```python
from build123d import *

# Parameters (mm, degrees)
SKETCH1_W                    = 125.73
SKETCH1_H                    = 76.2
BASE_FLANGE1_DEPTH           = 1.2192
EDGE_FLANGE1_STRIP_W         = 7.4168
EDGE_FLANGE1_STRIP_H         = 1.2192
EDGE_FLANGE1_STRIP_CUT_DEPTH = 76.2
EDGE_FLANGE1_DEPTH           = 76.2
EDGE_FLANGE2_STRIP_W         = 7.4168
EDGE_FLANGE2_STRIP_H         = 1.2192
EDGE_FLANGE2_STRIP_CUT_DEPTH = 123.2408
EDGE_FLANGE2_DEPTH           = 123.2408
EDGE_FLANGE3_STRIP_W         = 7.4168
EDGE_FLANGE3_STRIP_H         = 1.2192
EDGE_FLANGE3_STRIP_CUT_DEPTH = 200.7108
EDGE_FLANGE3_DEPTH           = 200.7108
BREAK_CORNER5_START          = -96.12466152
BREAK_CORNER5_OUTLINE_W      = 143.62455456
BREAK_CORNER5_OUTLINE_H      = 4
BREAK_CORNER5_DEPTH          = 7.220125921
BREAK_CORNER5_START_2        = 38.579180296
BREAK_CORNER5_2_OUTLINE_W    = 8.37544544
BREAK_CORNER5_2_OUTLINE_H    = 4
BREAK_CORNER5_2_DEPTH        = 14.440251843
BREAK_CORNER6_START          = -96.12466152
BREAK_CORNER6_OUTLINE_W      = 88.7601302
BREAK_CORNER6_OUTLINE_H      = 4
BREAK_CORNER6_DEPTH          = 7.220125921
BREAK_CORNER6_START_2        = -16.200382042
BREAK_CORNER6_2_OUTLINE_W    = 8.2398698
BREAK_CORNER6_2_OUTLINE_H    = 4
BREAK_CORNER6_2_DEPTH        = 14.440251842


# Read off the part's stored shape, not the designer's step: Break-Corner5, Break-Corner6
# Sheet-metal steps are written as plain solids
with BuildPart() as part:
    # Sketch1 → Base-Flange1 (new body)
    with BuildSketch(Plane(origin=(0, 0, 0), x_dir=(0, 0, -1), z_dir=(1, 0, 0))):
        with Locations((62.865, 38.1)):
            Rectangle(SKETCH1_W, SKETCH1_H)
    extrude(amount=-BASE_FLANGE1_DEPTH)

    # Edge-Flange1 strip (across the edge) → Edge-Flange1 strip cut (cut)
    with BuildSketch(Plane(origin=(0, 0, -125.73), x_dir=(0, 0, 1), z_dir=(0, 1, 0))):
        with Locations((-1.2192, -0.6096)):
            Rectangle(EDGE_FLANGE1_STRIP_W, EDGE_FLANGE1_STRIP_H)
    extrude(amount=EDGE_FLANGE1_STRIP_CUT_DEPTH, mode=Mode.SUBTRACT)

    # Edge-Flange1 section (across the edge) → Edge-Flange1 (add)
    with BuildSketch(Plane(origin=(0, 0, -125.73), x_dir=(0, 0, 1), z_dir=(0, 1, 0))):
        with BuildLine():
            Line((0, 1.27), (0, 201.9808))
            Line((0, 201.9808), (1.2192, 201.9808))
            Line((1.2192, 201.9808), (1.2192, 1.27))
            ThreePointArc((1.2192, 1.27), (1.591174388, 0.371974388), (2.4892, 0))
            Line((2.4892, 0), (2.4892, -1.2192))
            ThreePointArc((2.4892, -1.2192), (0.7290698, -0.4901302), (0, 1.27))
        make_face()
    extrude(amount=EDGE_FLANGE1_DEPTH)

    # Edge-Flange2 strip (across the edge) → Edge-Flange2 strip cut (cut)
    with BuildSketch(Plane(origin=(-1.2192, 0, -123.2408), x_dir=(0, 1, 0), z_dir=(0, 0, 1))):
        with Locations((-1.2192, -0.6096)):
            Rectangle(EDGE_FLANGE2_STRIP_W, EDGE_FLANGE2_STRIP_H)
    extrude(amount=EDGE_FLANGE2_STRIP_CUT_DEPTH, mode=Mode.SUBTRACT)

    # Edge-Flange2 section (across the edge) → Edge-Flange2 (add)
    with BuildSketch(Plane(origin=(-1.2192, 0, -123.2408), x_dir=(0, 1, 0), z_dir=(0, 0, 1))):
        with BuildLine():
            Line((0, 1.27), (0, 11.4808))
            Line((0, 11.4808), (1.2192, 11.4808))
            Line((1.2192, 11.4808), (1.2192, 1.27))
            ThreePointArc((1.2192, 1.27), (1.591174388, 0.371974388), (2.4892, 0))
            Line((2.4892, 0), (2.4892, -1.2192))
            ThreePointArc((2.4892, -1.2192), (0.7290698, -0.4901302), (0, 1.27))
        make_face()
    extrude(amount=EDGE_FLANGE2_DEPTH)

    # Edge-Flange3 strip (across the edge) → Edge-Flange3 strip cut (cut)
    with BuildSketch(Plane(origin=(201.9808, 0, -125.73), x_dir=(0, 1, 0), z_dir=(-1, 0, 0))):
        with Locations((-1.2192, -0.6096)):
            Rectangle(EDGE_FLANGE3_STRIP_W, EDGE_FLANGE3_STRIP_H)
    extrude(amount=EDGE_FLANGE3_STRIP_CUT_DEPTH, mode=Mode.SUBTRACT)

    # Edge-Flange3 section (across the edge) → Edge-Flange3 (add)
    with BuildSketch(Plane(origin=(201.9808, 0, -125.73), x_dir=(0, 1, 0), z_dir=(-1, 0, 0))):
        with BuildLine():
            Line((0, 1.27), (0, 11.4808))
            Line((0, 11.4808), (1.2192, 11.4808))
            Line((1.2192, 11.4808), (1.2192, 1.27))
            ThreePointArc((1.2192, 1.27), (1.591174388, 0.371974388), (2.4892, 0))
            Line((2.4892, 0), (2.4892, -1.2192))
            ThreePointArc((2.4892, -1.2192), (0.7290698, -0.4901302), (0, 1.27))
        make_face()
    extrude(amount=EDGE_FLANGE3_DEPTH)

    # Break-Corner5 outline → Break-Corner5 (cut)
    with BuildSketch(Plane(origin=(0, 0, 0), x_dir=(0.707106781186546, 0, -0.707106781186549), z_dir=(0.707106781186549, 0, 0.707106781186546)).offset(BREAK_CORNER5_START)):
        with Locations((160.81227728, 1)):
            Rectangle(BREAK_CORNER5_OUTLINE_W, BREAK_CORNER5_OUTLINE_H)
    extrude(amount=BREAK_CORNER5_DEPTH, mode=Mode.SUBTRACT)

    # Break-Corner5 2 outline → Break-Corner5 2 (cut)
    with BuildSketch(Plane(origin=(0, 0, 0), x_dir=(0.707106781186546, 0, -0.707106781186549), z_dir=(0.707106781186549, 0, 0.707106781186546)).offset(BREAK_CORNER5_START_2)):
        with Locations((236.81227728, 1)):
            Rectangle(BREAK_CORNER5_2_OUTLINE_W, BREAK_CORNER5_2_OUTLINE_H)
    extrude(amount=BREAK_CORNER5_2_DEPTH, mode=Mode.SUBTRACT)

    # Break-Corner6 outline → Break-Corner6 (cut)
    with BuildSketch(Plane(origin=(0, 0, 0), x_dir=(0.7071067811865471, 0, -0.707106781186548), z_dir=(0.707106781186548, 0, 0.707106781186547)).offset(BREAK_CORNER6_START)):
        with Locations((42.6199349, 1)):
            Rectangle(BREAK_CORNER6_OUTLINE_W, BREAK_CORNER6_OUTLINE_H)
    extrude(amount=BREAK_CORNER6_DEPTH, mode=Mode.SUBTRACT)

    # Break-Corner6 2 outline → Break-Corner6 2 (cut)
    with BuildSketch(Plane(origin=(0, 0, 0), x_dir=(0.7071067811865471, 0, -0.707106781186548), z_dir=(0.707106781186548, 0, 0.707106781186547)).offset(BREAK_CORNER6_START_2)):
        with Locations((-5.8800651, 1)):
            Rectangle(BREAK_CORNER6_2_OUTLINE_W, BREAK_CORNER6_2_OUTLINE_H)
    extrude(amount=BREAK_CORNER6_2_DEPTH, mode=Mode.SUBTRACT)


solid = part.part
```
The model under review builds one solid part; all positions refer to its coordinate system, in mm. A direction names the side the tool comes from. Coordinates: 2 decimals unless noted, no trailing zeros. Write each loop counter-clockwise with the first axis right and the second up, starting at its lowest first coordinate (ties: lowest second). Pieces come first, ordered by that corner, then holes.
1) Machinability: for faces 1 (the face through (-8, 0, -62)), 2 (the face through (103, 39, -124.511)), 3 (the face through (-1.219, 40, -61)), 4 (the face through (100, 39, -125.73)), which of the approach directions +Z, -Z, +X, -X, +Y, -Y give a long, thin tool a straight path to every point of the face, cutting with its end or side? Answer none if there is none.
2) Clearance check with flat-ended pins moving along their axes: pin 1 Ø1.4 at (y, z) = (1.5, -126) entering from -X; pin 2 Ø4 at (y, z) = (34, -43.5) entering from +X; pin 3 Ø10 at (y, z) = (65, -95) entering from -X; pin 4 Ø1.3 at (x, y) = (-0.5, 1) entering from +Z. State where each tip first meets the part, or that it passes through.
3) We need section B-B on y = 47. State the section outline as (x, z) points.
4) We need section A-A on z = -18. State the section outline as (x, y) points.
5) To check wall thickness, follow probe 1 along X at (y, z) = (8.5, -70.5); probe 2 along Z at (x, y) = (21, 13); probe 3 along Y at (x, z) = (89.5, -130). State the ranges of each line that lie inside material, in increasing order.
Answer list:
1. face 1: +Z, -Z, +X, -X, -Y
1. face 2: +Z, +X, +Y, -Y
1. face 3: +Z, -Z, -X, +Y
1. face 4: -Z, +X, -X, +Y
2. pin 1: stops at x = -0.13
2. pin 2: stops at x = 0
2. pin 3: stops at x = -1.22
2. pin 4: stops at z = 0
3. outline: (-1.22, -123.24) arc R2.49 ccw to (1.27, -125.73) - (201.98, -125.73) - (201.98, -124.51) - (1.27, -124.51) arc R1.27 cw to (0, -123.24) - (0, 0) - (-1.22, 0) - close
4. outline: (-12.7, 0) - (-2.49, 0) arc R2.49 ccw to (0, 2.49) - (0, 76.2) - (-1.22, 76.2) - (-1.22, 2.49) arc R1.27 cw to (-2.49, 1.22) - (-12.7, 1.22) - close
5. probe 1: x = -1.22 to 0
5. probe 2: z = -125.73 to -124.51
5. probe 3: y = 0 to 1.22
